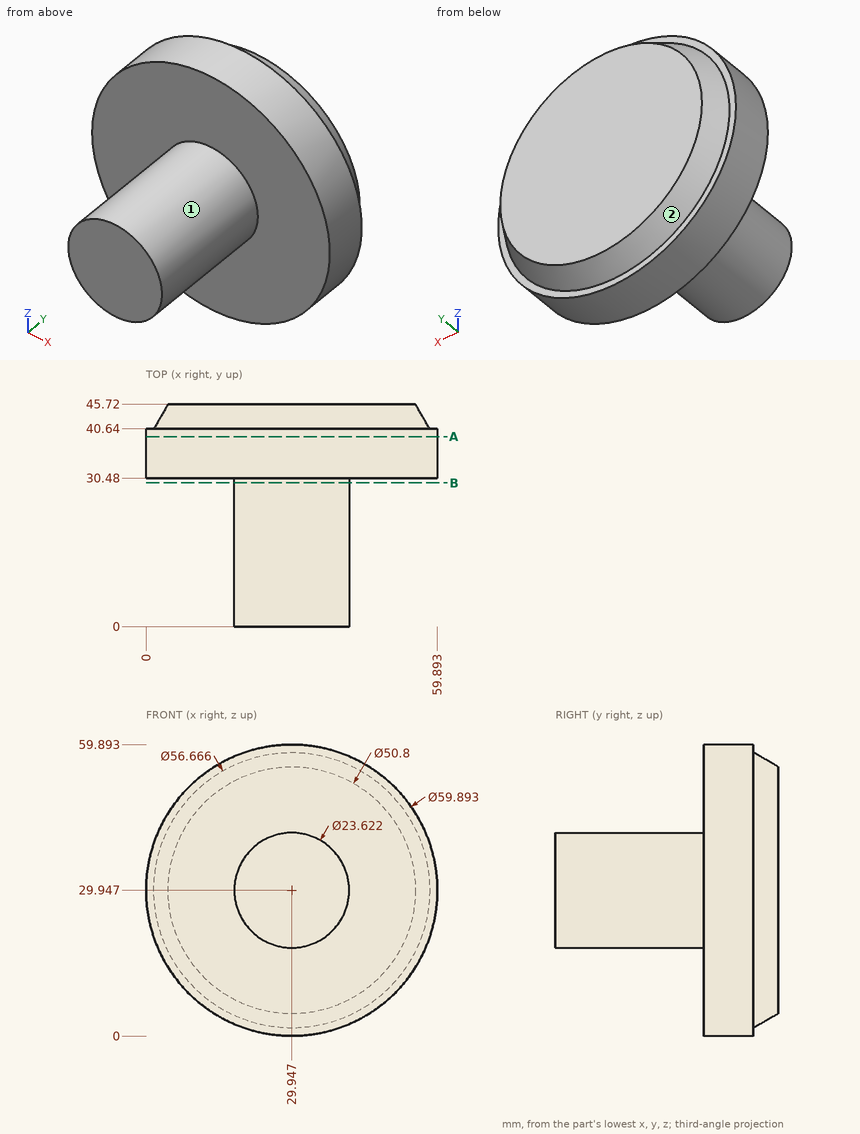
Part print with two shaded views. Sizes in mm from the minimum x, y, z corner. A direction names the side the tool comes from. Round coordinates to 2 decimals unless told otherwise and drop trailing zeros. Loops run counter-clockwise (first coordinate to the right, second up) from the corner with the lowest first, then second, coordinate; pieces in that order, holes last. Notation, with made-up numbers: M 75.25,13 L 133.25,13 A28 ccw 133.25,38 Z; hole C 18,16.5 d7. An arc over 180 degrees is marked long. Put each result on its own line as item: value. Start each with the question number.
Item 1: 3-axis set-ups, long thin cutter, end or side, ignore diameter. For the marked faces 1 and 2: which of +Z, -Z, +X, -X, +Y, -Y reach the whole face in a straight line?
Item 2: Cut at A-A (y = 39). List the corners of the cut face in (x, z), then the cut area to 3 significant figures.
Item 3: Drop flat-ended pins along their axis: P1, Ø8, axis at y = 41, z = 9, coming from the +X side (1 decimal); P2, Ø5, axis at y = 36, z = 41, coming from the -X side; P3, Ø8, axis at y = 30.5, z = 25.5, coming from the -X side. Give the stop position or say it passes through.
Item 4: Cut at B-B (y = 29.5). List the corners of the cut face in (x, z).
Item 5: Drill centre lines: line 1 along Y through (x, z) = (26, 8); line 2 along Y through (x, z) = (43, 56); line 3 along Z through (x, y) = (30.5, 40) (1 decimal). Where is each one in solid material? Low to high.
Answer block:
1. face 1: -Y
1. face 2: +Y
2. outline: C 29.95,29.95 d59.89
2. area: 2,820 mm2
3. P1: x = 54.6
3. P2: x = 1.25
3. P3: x = 0
4. outline: C 29.95,29.95 d23.62
5. line 1: 30.48 to 45.72
5. line 2: 30.48 to 40.64
5. line 3: 0 to 59.9
